Geometry: final body of the model. Coordinates: model frame, mm. Face numbers are marked on the shaded views. Give positions to 0.01 mm unless a question says otherwise; leave off trailing zeros. Write each loop counter-clockwise with the first axis right and the second up, starting at its lowest first coordinate (ties: lowest second). Pieces come first, ordered by that corner, then holes.
```python
from build123d import *

# Parameters (mm, degrees)
F1_DEPTH = 19
F0_R     = 2.25
F0_W     = 54
F0_H     = 54
F0_R_2   = 36
F0_R_3   = 2
F0_R_4   = 21
F2_DEPTH = 15
F3_DEPTH = 12
F4_R     = 5


with BuildPart() as f1:
    # F0 (on Front) → F1 (new body)
    with BuildSketch(Plane.XZ):
        with BuildLine():
            Line((-41.5, -82.5), (41.5, -82.5))
            ThreePointArc((41.5, -82.5), (43.267767, -81.767767), (44, -80))
            Line((44, -80), (44, 80))
            ThreePointArc((44, 80), (43.267767, 81.767767), (41.5, 82.5))
            Line((41.5, 82.5), (-41.5, 82.5))
            ThreePointArc((-41.5, 82.5), (-43.267767, 81.767767), (-44, 80))
            Line((-44, 80), (-44, -80))
            ThreePointArc((-44, -80), (-43.267767, -81.767767), (-41.5, -82.5))
        make_face()
        with BuildLine():
            ThreePointArc((-41.5, -80.5), (-41.853553, -80.353553), (-42, -80))
            Line((-42, -80), (-42, 80))
            ThreePointArc((-42, 80), (-41.853553, 80.353553), (-41.5, 80.5))
            Line((-41.5, 80.5), (41.5, 80.5))
            ThreePointArc((41.5, 80.5), (41.853553, 80.353553), (42, 80))
            Line((42, 80), (42, -80))
            ThreePointArc((42, -80), (41.853553, -80.353553), (41.5, -80.5))
            Line((41.5, -80.5), (-41.5, -80.5))
        make_face(mode=Mode.SUBTRACT)
    extrude(amount=F1_DEPTH)

    # F0 (on Front) → F2 (join)
    with BuildSketch(Plane.XZ):
        with BuildLine():
            Line((-42, 80), (-42, -80))
            ThreePointArc((-42, -80), (-41.853553, -80.353553), (-41.5, -80.5))
            Line((-41.5, -80.5), (41.5, -80.5))
            ThreePointArc((41.5, -80.5), (41.853553, -80.353553), (42, -80))
            Line((42, -80), (42, 80))
            ThreePointArc((42, 80), (41.853553, 80.353553), (41.5, 80.5))
            Line((41.5, 80.5), (-41.5, 80.5))
            ThreePointArc((-41.5, 80.5), (-41.853553, 80.353553), (-42, 80))
        make_face()
        with BuildLine():
            ThreePointArc((-37.677051, 77.5), (-36, 78.25), (-34.322949, 77.5))
            Line((-34.322949, 77.5), (34.322949, 77.5))
            ThreePointArc((34.322949, 77.5), (36, 78.25), (37.677051, 77.5))
            Line((37.677051, 77.5), (39, 77.5))
            Line((39, 77.5), (39, -77.5))
            Line((39, -77.5), (37.677051, -77.5))
            ThreePointArc((37.677051, -77.5), (36, -78.25), (34.322949, -77.5))
            Line((34.322949, -77.5), (-34.322949, -77.5))
            ThreePointArc((-34.322949, -77.5), (-36, -78.25), (-37.677051, -77.5))
            Line((-37.677051, -77.5), (-39, -77.5))
            Line((-39, -77.5), (-39, 77.5))
            Line((-39, 77.5), (-37.677051, 77.5))
        make_face(mode=Mode.SUBTRACT)
        with BuildLine():
            ThreePointArc((-34.322949, 77.5), (-33.898112, 76.80285), (-33.75, 76))
            ThreePointArc((-33.75, 76), (-36.80285, 73.898112), (-37.677051, 77.5))
            Line((-37.677051, 77.5), (-39, 77.5))
            Line((-39, 77.5), (-39, -77.5))
            Line((-39, -77.5), (-37.677051, -77.5))
            ThreePointArc((-37.677051, -77.5), (-36.80285, -73.898112), (-33.75, -76))
            ThreePointArc((-33.75, -76), (-33.898112, -76.80285), (-34.322949, -77.5))
            Line((-34.322949, -77.5), (34.322949, -77.5))
            ThreePointArc((34.322949, -77.5), (35.19715, -73.898112), (38.25, -76))
            ThreePointArc((38.25, -76), (38.101888, -76.80285), (37.677051, -77.5))
            Line((37.677051, -77.5), (39, -77.5))
            Line((39, -77.5), (39, 77.5))
            Line((39, 77.5), (37.677051, 77.5))
            ThreePointArc((37.677051, 77.5), (38.101888, 76.80285), (38.25, 76))
            ThreePointArc((38.25, 76), (35.19715, 73.898112), (34.322949, 77.5))
            Line((34.322949, 77.5), (-34.322949, 77.5))
        make_face()
        with Locations((-36, -4)):
            Circle(F0_R, mode=Mode.SUBTRACT)
        with Locations((0, -40)):
            Rectangle(F0_W, F0_H, mode=Mode.SUBTRACT)
        with Locations((36, -4)):
            Circle(F0_R, mode=Mode.SUBTRACT)
        with Locations((-36, 4)):
            Circle(F0_R, mode=Mode.SUBTRACT)
        with Locations((0, 40)):
            Circle(F0_R_2, mode=Mode.SUBTRACT)
        with Locations((36, 4)):
            Circle(F0_R, mode=Mode.SUBTRACT)
        with Locations((0, -40)):
            Rectangle(F0_W, F0_H)
        with Locations((-19.79899, -59.79899)):
            Circle(F0_R_3, mode=Mode.SUBTRACT)
        with Locations((-19.79899, -20.20101)):
            Circle(F0_R_3, mode=Mode.SUBTRACT)
        with Locations((19.79899, -59.79899)):
            Circle(F0_R_3, mode=Mode.SUBTRACT)
        with Locations((0, -40)):
            Circle(F0_R_4, mode=Mode.SUBTRACT)
        with Locations((19.79899, -20.20101)):
            Circle(F0_R_3, mode=Mode.SUBTRACT)
    extrude(amount=F2_DEPTH)

    # F0 (on Front) → F3 (cut)
    with BuildSketch(Plane.XZ):
        with Locations((0, -40)):
            Rectangle(F0_W, F0_H)
        with Locations((-19.79899, -59.79899)):
            Circle(F0_R_3, mode=Mode.SUBTRACT)
        with Locations((-19.79899, -20.20101)):
            Circle(F0_R_3, mode=Mode.SUBTRACT)
        with Locations((19.79899, -59.79899)):
            Circle(F0_R_3, mode=Mode.SUBTRACT)
        with Locations((0, -40)):
            Circle(F0_R_4, mode=Mode.SUBTRACT)
        with Locations((19.79899, -20.20101)):
            Circle(F0_R_3, mode=Mode.SUBTRACT)
    extrude(amount=F3_DEPTH, mode=Mode.SUBTRACT)

    # F4
    f4_edges = [f1.edges().sort_by_distance(p)[0] for p in [
        (-36, -15, 40),
    ]]
    fillet(f4_edges, radius=F4_R)


solid = f1.part
```
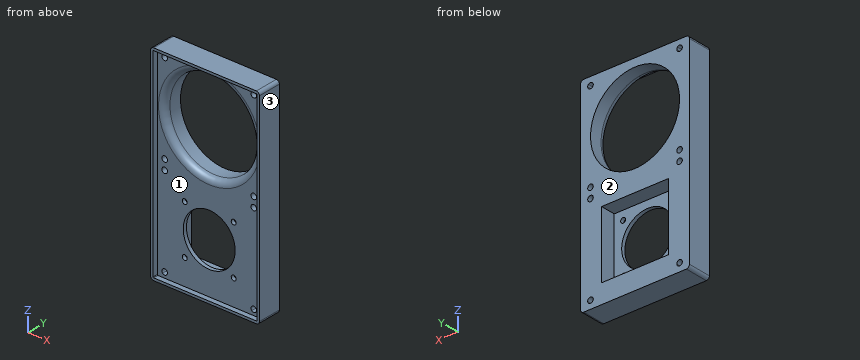
Item 1: Section B-B, the plane y = -8. State how many separate pieces and enclosed holes the cut face has, plus the area to 3 significant figures.
Found:
separate pieces: 1
enclosed holes: 10
area: 7,400 mm2
Item 2: Pull-direction query (X, two-part tool) for the marked faces 1, 2 and 3; classes: +X half, -X half, draft (parallel to the pull), parting line (faces both ways), or undercut.
Found:
face 1: undercut
face 2: draft
face 3: +X half
Item 3: Section A-A, the plane z = 40. Return the cut outline in (x, y).
Found:
outline: (-44, -19) - (-42, -19) - (-42, -15) - (-41, -15) arc R5 ccw to (-36, -10) - (-36, 0) - (-44, 0) - close; (36, -10) arc R5 ccw to (41, -15) - (42, -15) - (42, -19) - (44, -19) - (44, 0) - (36, 0) - close
Item 4: Pin query (flat end, axial travel): pin 1 Ø6 at (x, z) = (36, -4) entering from -Y; pin 2 Ø6 at (x, z) = (36, 76) entering from +Y. Return the tip coordinate at first contact, or that it passes through.
Found:
pin 1: stops at y = -15
pin 2: stops at y = 0
Item 5: Section C-C, the plane z = -16.5. Return the cut outline in (x, y).
Found:
outline: (-44, -19) - (-42, -19) - (-42, -15) - (42, -15) - (42, -19) - (44, -19) - (44, 0) - (27, 0) - (27, -12) - (-27, -12) - (-27, 0) - (-44, 0) - close
Item 6: Line query: L1, parallel to X at y = -7.5, z = -76; L2, parallel to Z at x = 25, y = -17.5; L3, parallel to Z at x = 0, y = -9.25. Output: solid intervals per line, ascending.
Found:
L1: x = -44 to -38.25, -33.75 to 33.75, 38.25 to 44
L2: z = -82.5 to -80.5, 80.5 to 82.5
L3: z = -82.5 to -67, -13 to 4, 76 to 82.5
